```python
from build123d import *

# Parameters (mm, degrees)
SKETCH1_R           = 1.7
BOSS_EXTRUDE1_DEPTH = 28.9
CUT_EXTRUDE1_REACH  = 33.757
SKETCH2_R           = 1.25
CUT_EXTRUDE2_DEPTH  = 3
SKETCH4_R           = 3.5
SKETCH4_R_2         = 2.5
BOSS_EXTRUDE2_DEPTH = 0.4
CUT_EXTRUDE3_START  = -3.5
SKETCH5_R           = 2.5
CUT_EXTRUDE3_DEPTH  = 3.5


with BuildPart() as part:
    # Sketch1 → Boss-Extrude1 (new body)
    with BuildSketch(Plane(origin=(0, 0, 0), x_dir=(1, 0, 0), z_dir=(0, 1, 0))):
        with BuildLine():
            Line((-9.7, 0), (9.7, 0))
            Line((9.7, 0), (9.7, -5.9))
            ThreePointArc((9.7, -5.9), (8.821320344, -8.021320344), (6.7, -8.9))
            Line((6.7, -8.9), (-6.7, -8.9))
            ThreePointArc((-6.7, -8.9), (-8.821320344, -8.021320344), (-9.7, -5.9))
            Line((-9.7, -5.9), (-9.7, 0))
        make_face()
        with Locations(Location((0, -2.23, 0), (0, 0, 270))):
            Circle(SKETCH1_R, mode=Mode.SUBTRACT)
    extrude(amount=BOSS_EXTRUDE1_DEPTH)

    # Cut-Extrude1: up to this face of the body (flat: up to its plane)
    cut_extrude1_end = Plane(part.part.faces().sort_by_distance((0, 14.45, 8.9))[0])
    # Sketch2 → Cut-Extrude1 (cut, up to the picked face)
    with BuildSketch(Plane(origin=(0, 0, 0), x_dir=(-1, 0, 0), z_dir=(0, 0, -1)), mode=Mode.PRIVATE) as cut_extrude1_sk1:
        with Locations((5.56, 25.044233664)):
            Circle(SKETCH2_R)
    cut_extrude1_tool1 = split(extrude(cut_extrude1_sk1.sketch, amount=-CUT_EXTRUDE1_REACH, mode=Mode.PRIVATE), bisect_by=cut_extrude1_end, keep=Keep.BOTH, mode=Mode.PRIVATE)
    # Sketch2 → Cut-Extrude1 (cut, up to the picked face)
    with BuildSketch(Plane(origin=(0, 0, 0), x_dir=(-1, 0, 0), z_dir=(0, 0, -1)), mode=Mode.PRIVATE) as cut_extrude1_sk2:
        with Locations((5.56, 3.855766336)):
            Circle(SKETCH2_R)
    cut_extrude1_tool2 = split(extrude(cut_extrude1_sk2.sketch, amount=-CUT_EXTRUDE1_REACH, mode=Mode.PRIVATE), bisect_by=cut_extrude1_end, keep=Keep.BOTH, mode=Mode.PRIVATE)
    # Sketch2 → Cut-Extrude1 (cut, up to the picked face)
    with BuildSketch(Plane(origin=(0, 0, 0), x_dir=(-1, 0, 0), z_dir=(0, 0, -1)), mode=Mode.PRIVATE) as cut_extrude1_sk3:
        with Locations((-5.56, 3.855766336)):
            Circle(SKETCH2_R)
    cut_extrude1_tool3 = split(extrude(cut_extrude1_sk3.sketch, amount=-CUT_EXTRUDE1_REACH, mode=Mode.PRIVATE), bisect_by=cut_extrude1_end, keep=Keep.BOTH, mode=Mode.PRIVATE)
    # Sketch2 → Cut-Extrude1 (cut, up to the picked face)
    with BuildSketch(Plane(origin=(0, 0, 0), x_dir=(-1, 0, 0), z_dir=(0, 0, -1)), mode=Mode.PRIVATE) as cut_extrude1_sk4:
        with Locations((-5.56, 25.044233664)):
            Circle(SKETCH2_R)
    cut_extrude1_tool4 = split(extrude(cut_extrude1_sk4.sketch, amount=-CUT_EXTRUDE1_REACH, mode=Mode.PRIVATE), bisect_by=cut_extrude1_end, keep=Keep.BOTH, mode=Mode.PRIVATE)
    add(cut_extrude1_tool1.solids().sort_by(Axis((-5.56, 25.044234, 0), (0, 0, 1)))[0], mode=Mode.SUBTRACT)
    add(cut_extrude1_tool2.solids().sort_by(Axis((-5.56, 3.855766, 0), (0, 0, 1)))[0], mode=Mode.SUBTRACT)
    add(cut_extrude1_tool3.solids().sort_by(Axis((5.56, 3.855766, 0), (0, 0, 1)))[0], mode=Mode.SUBTRACT)
    add(cut_extrude1_tool4.solids().sort_by(Axis((5.56, 25.044234, 0), (0, 0, 1)))[0], mode=Mode.SUBTRACT)

    # Sketch3 → Cut-Extrude2 (cut)
    with BuildSketch(Plane.XY.offset(8.9)):
        with BuildLine():
            Line((5.56, 7.711532672), (9.7, 7.711532672))
            Line((9.7, 7.711532672), (9.7, 0))
            Line((9.7, 0), (1.7, 0))
            Line((1.7, 0), (1.704233664, 3.855766336))
            ThreePointArc((1.704233664, 3.855766336), (2.833561477, 6.582204859), (5.56, 7.711532672))
        make_face()
        with BuildLine():
            Line((5.56, 21.188467328), (9.7, 21.188467328))
            Line((9.7, 21.188467328), (9.7, 28.9))
            Line((9.7, 28.9), (1.7, 28.9))
            Line((1.7, 28.9), (1.704233664, 25.044233664))
            ThreePointArc((1.704233664, 25.044233664), (2.833561477, 22.317795141), (5.56, 21.188467328))
        make_face()
        with BuildLine():
            Line((-1.704233664, 3.855766336), (-1.7, 0))
            Line((-1.7, 0), (-9.7, 0))
            Line((-9.7, 0), (-9.7, 7.711532672))
            Line((-9.7, 7.711532672), (-5.56, 7.711532672))
            ThreePointArc((-5.56, 7.711532672), (-2.833561477, 6.582204859), (-1.704233664, 3.855766336))
        make_face()
        with BuildLine():
            Line((-9.7, 28.9), (-9.7, 21.188467328))
            Line((-9.7, 21.188467328), (-5.56, 21.188467328))
            ThreePointArc((-5.56, 21.188467328), (-2.833561477, 22.317795141), (-1.704233664, 25.044233664))
            Line((-1.704233664, 25.044233664), (-1.7, 28.9))
            Line((-1.7, 28.9), (-9.7, 28.9))
        make_face()
    extrude(amount=-CUT_EXTRUDE2_DEPTH, mode=Mode.SUBTRACT)

    # Sketch4 → Boss-Extrude2 (add)
    with BuildSketch(Plane(origin=(0, 0, 0), x_dir=(-1, 0, 0), z_dir=(0, 0, -1))):
        with Locations(Location((0, 14.45, 0), (0, 0, 180))):
            Circle(SKETCH4_R)
        with Locations((0, 14.45)):
            Circle(SKETCH4_R_2, mode=Mode.SUBTRACT)
    extrude(amount=BOSS_EXTRUDE2_DEPTH)

    # Sketch5 → Cut-Extrude3 (cut)
    with BuildSketch(Plane(origin=(0, 0, -0.4), x_dir=(-1, 0, 0), z_dir=(0, 0, -1)).offset(CUT_EXTRUDE3_START)):
        with Locations(Location((0, 14.45, 0), (0, 0, 234.253121961))):
            Circle(SKETCH5_R)
    extrude(amount=CUT_EXTRUDE3_DEPTH, mode=Mode.SUBTRACT)


solid = part.part
```
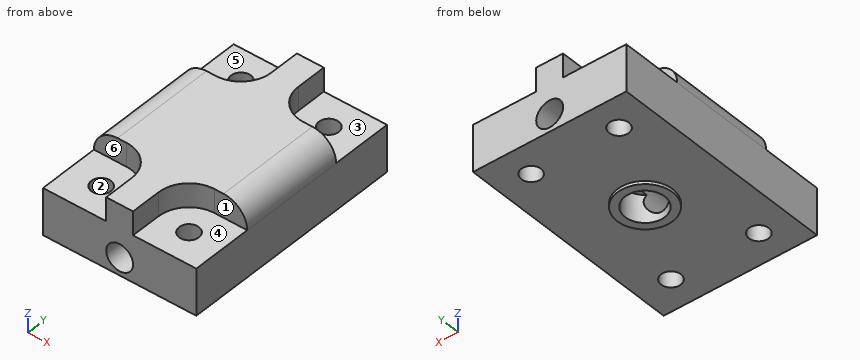
Here's how the part is built. I have some questions about the finished solid (model axes, mm). Face numbers are marked on the shaded views. A direction names the side the tool comes from. Give positions to 0.01 mm unless a question says otherwise; leave off trailing zeros. Loops run counter-clockwise (first coordinate to the right, second up) from the corner with the lowest first, then second, coordinate; pieces in that order, holes last. Notation, with made-up numbers: M 49.5,50.25 L 59.5,50.25 A18 cw 59.5,79.25 Z; hole C -2,7 d2. An arc over 180 degrees is marked long. Return JSON: item names as keys, results as strings.
Item 1: Imagine slicing it at A-A on z = 2.23. List the corners of the cut face in (x, y) for me, then the cut area to 3 significant figures.
A:
{"outline": "M -9.7,0 L -1.7,0 L -1.7,12.62 A2.5 cw -1.7,16.28 L -1.7,28.9 L -9.7,28.9 Z; M 1.7,0 L 9.7,0 L 9.7,28.9 L 1.7,28.9 L 1.7,16.28 A2.5 cw 1.7,12.62 Z; hole C -5.56,3.86 d2.5; hole C -5.56,25.04 d2.5; hole C 5.56,3.86 d2.5; hole C 5.56,25.04 d2.5", "area": "439 mm^2"}
Item 2: I'm going to push flat-ended pins straight in: pin 1 Ø1.5 at (x, y) = (5.56, 25.04) entering from +Z; pin 2 Ø3 at (x, y) = (-5.56, 25.04) entering from +Z; pin 3 Ø3.5 at (x, z) = (-8.5, 8) entering from -Y; pin 4 Ø4 at (x, y) = (4.5, 25.5) entering from -Z. Where does each tip first touch, or does it pass through?
A:
{"pin 1": "passes through", "pin 2": "stops at z = 5.9", "pin 3": "stops at y = 7.71", "pin 4": "stops at z = 0"}
Item 3: Please list where these lines run through material, in increasing order: line 1 (X direction, y = 17.5, z = 2.23); line 2 (Y direction, x = -5, z = 4.5); line 3 (Z direction, x = 6, y = 23.5).
A:
{"line 1": "x = -9.7 to -1.7, 1.7 to 9.7", "line 2": "y = 0 to 2.74, 4.97 to 23.93, 26.16 to 28.9", "line 3": "z = 0 to 5.9"}
Item 4: Imagine slicing it at B-B on y = 14.45. List the corners of the cut face in (x, z) for me, then the cut area to 3 significant figures.
A:
{"outline": "M -9.7,0 L -3.5,0 L -3.5,-0.4 L -2.5,-0.4 L -2.5,3.1 L -1.46,3.1 A1.7 cw 1.46,3.1 L 2.5,3.1 L 2.5,-0.4 L 3.5,-0.4 L 3.5,0 L 9.7,0 L 9.7,5.9 A3 ccw 6.7,8.9 L -6.7,8.9 A3 ccw -9.7,5.9 Z", "area": "152 mm^2"}
Item 5: Imagine slicing it at D-D on x = -8.5. List the corners of the cut face in (y, z) for me.
A:
{"outline": "M 0,0 L 28.9,0 L 28.9,5.9 L 21.19,5.9 L 21.19,8.3 L 7.71,8.3 L 7.71,5.9 L 0,5.9 Z"}
Item 6: Imagine slicing it at C-C on x = 0. List the corners of the cut face in (y, z) for me, then the cut area to 3 significant figures.
A:
{"outline": "M 0,0 L 10.95,0 L 10.95,-0.4 L 11.95,-0.4 L 11.95,0.53 L 0,0.53 Z; M 0,3.93 L 28.9,3.93 L 28.9,8.9 L 0,8.9 Z; M 16.95,-0.4 L 17.95,-0.4 L 17.95,0 L 28.9,0 L 28.9,0.53 L 16.95,0.53 Z", "area": "157 mm^2"}
Item 7: Thinking about a two-plate mould opening in Y: for the marked faces 1, 2 and 3, which applies, released by +Y, released by -Y, zero draft, split by the parting line, or undercut?
A:
{"face 1": "released by -Y", "face 2": "undercut", "face 3": "zero draft"}
Item 8: On a 3-axis mill with a long thin cutter (end or side, diameter ignored), from which of +Z, -Z, +X, -X, +Y, -Y can I reach the whole of each face in a straight line? I mean the marked faces 4, 5 and 6. Say none if no direction works.
A:
{"face 4": "+Z, +X, -Y", "face 5": "+Z, -X, +Y", "face 6": "+Z, -X, -Y"}
